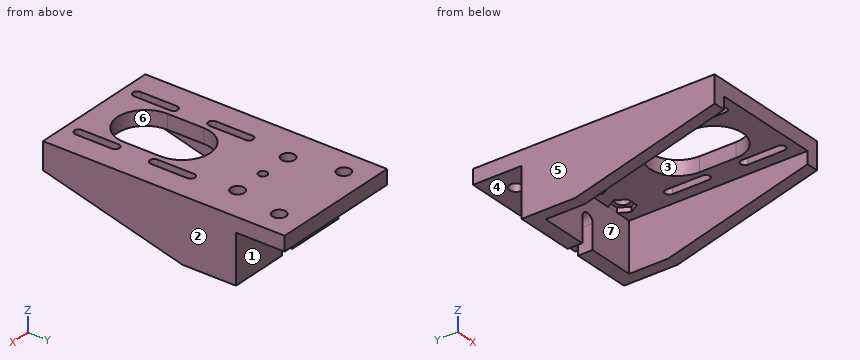
from build123d import *

# Parameters (mm, degrees)
SKETCH_W        = 54.3
SKETCH_H        = 57.3
PAD_DEPTH       = 6
SKETCH001_W     = 54.3
SKETCH001_H     = 26
PAD001_DEPTH    = 42
SKETCH002_W     = 20
SKETCH002_H     = 20
POCKET_DEPTH    = 54.301
PAD002_DEPTH    = 5
SKETCH004_R     = 2.75
POCKET001_DEPTH = 6.001
SKETCH005_W     = 44.3
SKETCH005_H     = 20
POCKET002_DEPTH = 16
SKETCH006_R     = 2.75
SKETCH006_R_2   = 1.75
POCKET003_DEPTH = 6.001
POCKET004_DEPTH = 2
POCKET005_DEPTH = 79.301


with BuildPart() as part:
    # Sketch → Pad (new body)
    with BuildSketch(Plane.XY):
        with Locations((0, -7.5)):
            Rectangle(SKETCH_W, SKETCH_H)
        with BuildLine():
            ThreePointArc((-13.75, 15.5), (-15.5, 17.25), (-17.25, 15.5))
            Line((-17.25, 15.5), (-17.25, 0.5))
            ThreePointArc((-17.25, 0.5), (-15.5, -1.25), (-13.75, 0.5))
            Line((-13.75, 0.5), (-13.75, 15.5))
        make_face(mode=Mode.SUBTRACT)
        with BuildLine():
            ThreePointArc((17.25, 15.5), (15.5, 17.25), (13.75, 15.5))
            Line((13.75, 15.5), (13.75, 0.5))
            ThreePointArc((13.75, 0.5), (15.5, -1.25), (17.25, 0.5))
            Line((17.25, 0.5), (17.25, 15.5))
        make_face(mode=Mode.SUBTRACT)
        with BuildLine():
            ThreePointArc((-13.75, -15.5), (-15.5, -13.75), (-17.25, -15.5))
            Line((-17.25, -15.5), (-17.25, -30.5))
            ThreePointArc((-17.25, -30.5), (-15.5, -32.25), (-13.75, -30.5))
            Line((-13.75, -30.5), (-13.75, -15.5))
        make_face(mode=Mode.SUBTRACT)
        with BuildLine():
            ThreePointArc((17.25, -15.5), (15.5, -13.75), (13.75, -15.5))
            Line((13.75, -15.5), (13.75, -30.5))
            ThreePointArc((13.75, -30.5), (15.5, -32.25), (17.25, -30.5))
            Line((17.25, -30.5), (17.25, -15.5))
        make_face(mode=Mode.SUBTRACT)
        with BuildLine():
            ThreePointArc((11.5, 0), (0, 11.5), (-11.5, 0))
            Line((-11.5, 0), (-11.5, -15))
            ThreePointArc((-11.5, -15), (0, -26.5), (11.5, -15))
            Line((11.5, -15), (11.5, 0))
        make_face(mode=Mode.SUBTRACT)
    extrude(amount=PAD_DEPTH)

    # Sketch001 (on Face1 of Pad) → Pad001 (join)
    with BuildSketch(Plane(origin=(0, 21.15, 0), x_dir=(-1, 0, 0), z_dir=(0, 1, 0))):
        with Locations((0, -7)):
            Rectangle(SKETCH001_W, SKETCH001_H)
    extrude(amount=PAD001_DEPTH)

    # Sketch002 (on Face26 of Pad001) → Pocket (cut, through all)
    with BuildSketch(Plane.YZ.offset(27.15)):
        with Locations((53.15, -10)):
            Rectangle(SKETCH002_W, SKETCH002_H)
    extrude(amount=-POCKET_DEPTH, mode=Mode.SUBTRACT)

    # Sketch003 (on Face3 of Pocket) → Pad002 (join)
    with BuildSketch(Plane(origin=(-27.15, 0, 0), x_dir=(0, -1, 0), z_dir=(-1, 0, 0))):
        Polygon((36.15, 0), (36.15, -5), (-21.15, -20), (-21.15, 0), align=None)
    pad002 = extrude(amount=-PAD002_DEPTH)

    # Mirrored: Pad002 across YZ
    add(pad002.mirror(Plane.YZ))

    # Sketch004 (on Face5 of Mirrored) → Pocket001 (cut, through all)
    with BuildSketch(Plane(origin=(0, 0, 0), x_dir=(1, 0, 0), z_dir=(0, 0, -1))):
        with Locations((-17.15, -53.15)):
            Circle(SKETCH004_R)
        with Locations((17.15, -53.15)):
            Circle(SKETCH004_R)
    extrude(amount=-POCKET001_DEPTH, mode=Mode.SUBTRACT)

    # Sketch005 (on Face5 of Pocket001) → Pocket002 (cut)
    with BuildSketch(Plane.XZ.offset(-21.15)):
        with Locations((0, -10)):
            Rectangle(SKETCH005_W, SKETCH005_H)
    extrude(amount=-POCKET002_DEPTH, mode=Mode.SUBTRACT)

    # Sketch006 (on Face5 of Pocket002) → Pocket003 (cut, through all)
    with BuildSketch(Plane(origin=(0, 0, 0), x_dir=(1, 0, 0), z_dir=(0, 0, -1))):
        with Locations((-13.4, -33.15)):
            Circle(SKETCH006_R)
        with Locations((13.4, -33.15)):
            Circle(SKETCH006_R)
        with Locations((0, -33.15)):
            Circle(SKETCH006_R_2)
    extrude(amount=-POCKET003_DEPTH, mode=Mode.SUBTRACT)

    # Sketch007 (on Face37 of Pocket003) → Pocket004 (cut)
    with BuildSketch(Plane(origin=(0, 0, 0), x_dir=(1, 0, 0), z_dir=(0, 0, -1))):
        Polygon((18.15, -33.15), (15.775, -29.036379), (11.025, -29.036379), (8.65, -33.15), (11.025, -37.263621), (15.775, -37.263621), align=None)
        Polygon((-8.65, -33.15), (-11.025, -29.036379), (-15.775, -29.036379), (-18.15, -33.15), (-15.775, -37.263621), (-11.025, -37.263621), align=None)
        Polygon((3.25, -33.15), (1.625, -30.335417), (-1.625, -30.335417), (-3.25, -33.15), (-1.625, -35.964583), (1.625, -35.964583), align=None)
    extrude(amount=-POCKET004_DEPTH, mode=Mode.SUBTRACT)

    # Sketch008 (on Face48 of Pocket004) → Pocket005 (cut, through all)
    with BuildSketch(Plane(origin=(0, 43.15, 0), x_dir=(-1, 0, 0), z_dir=(0, 1, 0))):
        with BuildLine():
            ThreePointArc((2.75, -10), (0, -7.25), (-2.75, -10))
            Line((-2.75, -10), (-2.75, -30))
            ThreePointArc((-2.75, -30), (0, -32.75), (2.75, -30))
            Line((2.75, -30), (2.75, -10))
        make_face()
    extrude(amount=-POCKET005_DEPTH, mode=Mode.SUBTRACT)


solid = part.part
Geometry check sheet. Reference: the model listing, model coordinates, mm. Face numbers are marked on the shaded views. A direction names the side the tool comes from. Round coordinates to 2 decimals unless told otherwise and drop trailing zeros. Write each loop counter-clockwise with the first axis right and the second up, starting at its lowest first coordinate (ties: lowest second). Pieces come first, ordered by that corner, then holes. Notation, with made-up numbers: (78.5, 68.25) - (97.5, 68.25) arc R26 ccw to (97.5, 103.25) - close; hole circle Ø3 at (35, 64.25). An arc over 180 degrees is marked (long way). One line per item, written item: value.
1. Scan lines: L1, parallel to Y at x = 0, z = 3.75; L2, parallel to X at y = 53.15, z = 1.4; L3, parallel to X at y = 33.15, z = 4.95. Record each from-to range of solid material in increasing order.
The answers:
L1: y = -36.15 to -26.5, 11.5 to 31.4, 34.9 to 63.15
L2: x = -27.15 to -19.9, -14.4 to 14.4, 19.9 to 27.15
L3: x = -27.15 to -16.15, -10.65 to -1.75, 1.75 to 10.65, 16.15 to 27.15
2. Cross-section at C-C on y = 23.5. Record the boundary of the cut face in (x, z), and give its area (3 significant figures).
The answers:
outline: (-27.15, -20) - (-22.15, -20) - (-22.15, 0) - (22.15, 0) - (22.15, -20) - (27.15, -20) - (27.15, 6) - (-27.15, 6) - close
area: 526 mm^2
3. Depth check by flat-ended pin: pin 1 Ø4.5 at (x, y) = (-17.15, 53.15) entering from -Z; pin 2 Ø6.5 at (x, y) = (-13.4, 33.15) entering from -Z; pin 3 Ø6 at (x, z) = (-6.5, -11) entering from -Y. Enter the tip coordinate at first touch or a pass-through.
The answers:
pin 1: passes through
pin 2: stops at z = 2
pin 3: stops at y = 37.15
4. Cross-section at B-B on z = -3. Record the boundary of the cut face in (x, y), and give its area (3 significant figures).
The answers:
outline: (-27.15, -36.15) - (-22.15, -36.15) - (-22.15, 37.15) - (22.15, 37.15) - (22.15, -36.15) - (27.15, -36.15) - (27.15, 43.15) - (-27.15, 43.15) - close
area: 1,060 mm^2
5. Mould release check, pull along Y, two halves, no side actions. Record for the marked faces 1, 2 and 3: released by +Y, released by -Y, zero draft, split by the parting line, or undercut.
The answers:
face 1: released by +Y
face 2: zero draft
face 3: undercut
6. Cross-section at D-D on x = 7. Record the boundary of the cut face in (y, z), and give its area (3 significant figures).
The answers:
outline: (-36.15, 0) - (-24.12, 0) - (-24.12, 6) - (-36.15, 6) - close; (9.12, 0) - (37.15, 0) - (37.15, -20) - (43.15, -20) - (43.15, 0) - (63.15, 0) - (63.15, 6) - (9.12, 6) - close
area: 516 mm^2
7. Set-up check for the marked faces 4, 5, 6 and 7: record each of +Z, -Z, +X, -X, +Y, -Y from which the full face is reachable in a straight line by a thin tool's end or side.
The answers:
face 4: -Z, +X, -X, +Y
face 5: +Z, -Z, -X, +Y, -Y
face 6: +Z, -Z
face 7: -Z, -Y
8. Cross-section at A-A on x = 0. Record the boundary of the cut face in (y, z).
The answers:
outline: (-36.15, 0) - (-26.5, 0) - (-26.5, 6) - (-36.15, 6) - close; (11.5, 0) - (30.34, 0) - (30.34, 2) - (31.4, 2) - (31.4, 6) - (11.5, 6) - close; (34.9, 2) - (35.96, 2) - (35.96, 0) - (37.15, 0) - (37.15, -7.25) - (43.15, -7.25) - (43.15, 0) - (63.15, 0) - (63.15, 6) - (34.9, 6) - close
